```python
from build123d import *

# Parameters (mm, degrees)
F0_W      = 104
F0_H      = 46
F1_DEPTH  = 5.8
F2_W      = 123
F2_H      = 9
F3_DEPTH  = 5.8
F4_R      = 1.25
F5_DEPTH  = 5.8
F6_R      = 1.25
F7_DEPTH  = 5.8
F8_W      = 100.1
F8_H      = 42.1
F9_DEPTH  = 1.8
F10_W     = 96
F10_H     = 38
F11_DEPTH = 4
F12_W     = 7.5
F12_H     = 7.5
F13_DEPTH = 4
F14_W     = 7.5
F14_H     = 7.5
F15_DEPTH = 4
F16_R     = 1.5
F17_DEPTH = 8
F18_R     = 1.5
F19_DEPTH = 8
F20_W     = 26
F20_H     = 26
F21_DEPTH = 4
F22_W     = 23
F22_H     = 23
F23_DEPTH = 3
F24_R     = 3
F25_R     = 4
F26_R     = 3
F27_R     = 3
F28_R     = 2
F29_R     = 1
F30_DEPTH = 1.8
F31_R     = 1
F32_DEPTH = 1.8
F33_R     = 1
F34_DEPTH = 1.8


with BuildPart() as f1:
    # F0 (on Top) → F1 (new body)
    with BuildSketch(Plane.XY):
        Rectangle(F0_W, F0_H)
    extrude(amount=F1_DEPTH)

    # F2 (on Top) → F3 (join)
    with BuildSketch(Plane.XY):
        with Locations((0, -18.5)):
            Rectangle(F2_W, F2_H)
    extrude(amount=F3_DEPTH)

    # F4 (on Top) → F5 (cut)
    with BuildSketch(Plane.XY):
        with Locations((-57.3, -18.8)):
            Circle(F4_R)
    extrude(amount=F5_DEPTH, mode=Mode.SUBTRACT)

    # F6 (on Top) → F7 (cut)
    with BuildSketch(Plane.XY):
        with Locations((57.3, -18.8)):
            Circle(F6_R)
    extrude(amount=F7_DEPTH, mode=Mode.SUBTRACT)

    # F8 (on face) → F9 (cut)
    with BuildSketch(Plane.XY.offset(5.8)):
        Rectangle(F8_W, F8_H)
    extrude(amount=-F9_DEPTH, mode=Mode.SUBTRACT)

    # F10 (on face) → F11 (cut)
    with BuildSketch(Plane.XY.offset(4)):
        Rectangle(F10_W, F10_H)
    extrude(amount=-F11_DEPTH, mode=Mode.SUBTRACT)

    # F12 (on Top) → F13 (join)
    with BuildSketch(Plane.XY):
        with Locations((-46.3, 17.3)):
            Rectangle(F12_W, F12_H)
    extrude(amount=F13_DEPTH)

    # F14 (on Top) → F15 (join)
    with BuildSketch(Plane.XY):
        with Locations((46.3, -17.3)):
            Rectangle(F14_W, F14_H)
    extrude(amount=F15_DEPTH)

    # F16 (on Top) → F17 (join)
    with BuildSketch(Plane.XY):
        with Locations((-46, 17)):
            Circle(F16_R)
    extrude(amount=F17_DEPTH)

    # F18 (on Top) → F19 (join)
    with BuildSketch(Plane.XY):
        with Locations((46, -17)):
            Circle(F18_R)
    extrude(amount=F19_DEPTH)

    # F20 (on Top) → F21 (join)
    with BuildSketch(Plane.XY):
        with Locations((-37.05, -8.05)):
            Rectangle(F20_W, F20_H)
    extrude(amount=F21_DEPTH)

    # F22 (on face) → F23 (cut)
    with BuildSketch(Plane.XY.offset(4)):
        with Locations((-36.55, -7.55)):
            Rectangle(F22_W, F22_H)
    extrude(amount=-F23_DEPTH, mode=Mode.SUBTRACT)

    # F24
    f24_edges = [f1.edges().sort_by_distance(p)[0] for p in [
        (-25.05, 3.95, 2.5),
    ]]
    fillet(f24_edges, radius=F24_R)

    # F25
    f25_edges = [f1.edges().sort_by_distance(p)[0] for p in [
        (-24.05, 4.95, 2),
    ]]
    fillet(f25_edges, radius=F25_R)

    # F26
    f26_edges = [f1.edges().sort_by_distance(p)[0] for p in [
        (-42.55, 13.55, 2),
    ]]
    fillet(f26_edges, radius=F26_R)

    # F27
    f27_edges = [f1.edges().sort_by_distance(p)[0] for p in [
        (42.55, -13.55, 2),
    ]]
    fillet(f27_edges, radius=F27_R)

    # F28
    f28_edges = [f1.edges().sort_by_distance(p)[0] for p in [
        (-61.5, -14, 2.9),
        (-61.5, -23, 2.9),
        (61.5, -23, 2.9),
        (61.5, -14, 2.9),
    ]]
    fillet(f28_edges, radius=F28_R)

    # F29 (on face) → F30 (cut)
    with BuildSketch(Plane.XY.offset(5.8)):
        with Locations((-50.05, 21.05)):
            Circle(F29_R)
    extrude(amount=-F30_DEPTH, mode=Mode.SUBTRACT)

    # F31 (on face) → F32 (cut)
    with BuildSketch(Plane.XY.offset(5.8)):
        with Locations((-50.05, -21.05)):
            Circle(F31_R)
    extrude(amount=-F32_DEPTH, mode=Mode.SUBTRACT)

    # F33 (on face) → F34 (cut)
    with BuildSketch(Plane.XY.offset(5.8)):
        with Locations((50.05, -21.05)):
            Circle(F33_R)
        with Locations((50.05, 21.05)):
            Circle(F33_R)
    extrude(amount=-F34_DEPTH, mode=Mode.SUBTRACT)


solid = f1.part
```
Can you work these out from the model? Positions are in its coordinate system, mm. A direction names the side the tool comes from. Give positions to 0.01 mm unless a question says otherwise; leave off trailing zeros. Write each loop counter-clockwise with the first axis right and the second up, starting at its lowest first coordinate (ties: lowest second). Pieces come first, ordered by that corner, then holes. Notation, with made-up numbers: (5.5, 28) - (36.5, 28) arc R24 ccw to (36.5, 39) - close; hole circle Ø3 at (27.25, 70). An arc over 180 degrees is marked (long way). Write item = value, one per line. Start each with the question number.
1. Imagine slicing it at B-B (y = 8.5). Please give me the cut outline in (x, z), and give its area (3 significant figures).
2. On a 3-axis mill with a long thin cutter (end or side, diameter ignored), from which of +Z, -Z, +X, -X, +Y, -Y can I reach the whole of each face in a straight line? I mean faces 4 (the face through (-56, -14, 3)), 5 (the face through (-43.45, 14.41, 2.03)), 6 (the face through (-25.91, 3.05, 2.48)). Say none if no direction works.
3. For pin 1 (1.2 mm diameter, centred on x = 50.05, y = -21.05, fed in from +Z); pin 2 (1 mm diameter, centred on x = 29.5, z = 6.5, fed in from -Y); pin 3 (3 mm diameter, centred on y = -14, z = 2, fed in from +X); pin 4 (3 mm diameter, centred on y = -2.5, z = 3, fed in from -X), each with a flat end and sliding along its axis, tell me the tip position at first contact or that it passes through.
4. Imagine slicing it at A-A (x = 57.3). Please give me the cut outline in (y, z).
5. Please list where these lines run through material, in increasing order: line 1 (X direction, y = -11, z = 2.5); line 2 (Y direction, x = 47, z = 4.25); line 3 (X direction, y = 5, z = 4.5).
6. Imagine slicing it at D-D (y = -9). Please give me the cut outline in (x, z), and give its area (3 significant figures).
7. Thinking about a two-plate mould opening in Y: for faces 1 (the face through (-46, 17, 8)), 2 (the face through (-24.05, -9, 2)), 3 (the face through (60.93, -14.6, 2.94)), which applies, released by +Y, released by -Y, zero draft, split by the parting line, or undercut?
8. Imagine slicing it at C-C (z = 2.75). Count the separate pieces of the cut face and the enclosed holes in it, and give its area (3 significant figures).
Worked answers:
q1.outline = (-52, 0) - (-48, 0) - (-48, 4) - (-50.05, 4) - (-50.05, 5.8) - (-52, 5.8) - close; (48, 0) - (52, 0) - (52, 5.8) - (50.05, 5.8) - (50.05, 4) - (48, 4) - close
q1.area = 39.0 mm2
q2.face_4 = +Z, -Z, -X, +Y
q2.face_5 = +Z, -Z
q2.face_6 = +Z
q3.pin_1 = 4
q3.pin_2 = through
q3.pin_3 = 61.44
q3.pin_4 = -52
q4.outline = (-23, 0) - (-20.05, 0) - (-20.05, 5.8) - (-23, 5.8) - close; (-17.55, 0) - (-14, 0) - (-14, 5.8) - (-17.55, 5.8) - close
q5.line_1 = -52 to -48.05, -25.05 to -24.05, 48 to 52
q5.line_2 = -23 to -21.05, -18.12 to -15.88, 21.05 to 23
q5.line_3 = -52 to -50.05, 50.05 to 52
q6.outline = (-52, 0) - (-24.05, 0) - (-24.05, 4) - (-25.05, 4) - (-25.05, 1) - (-48.05, 1) - (-48.05, 4) - (-50.05, 4) - (-50.05, 5.8) - (-52, 5.8) - close; (48, 0) - (52, 0) - (52, 5.8) - (50.05, 5.8) - (50.05, 4) - (48, 4) - close
q6.area = 65.8 mm2
q7.face_1 = zero draft
q7.face_2 = undercut
q7.face_3 = released by +Y
q8.separate_pieces = 1
q8.enclosed_holes = 4
q8.area = 1,390 mm2
